from build123d import *

# Parameters (mm, degrees)
SKETCH1_W           = 88.9
SKETCH1_H           = 12.7
BOSS_EXTRUDE1_DEPTH = 6.35
SKETCH2_W           = 14.725
SKETCH2_H           = 6.326510552
SKETCH2_W_2         = 15.361563021
SKETCH2_H_2         = 6.35
BOSS_EXTRUDE2_DEPTH = 19.05
CUT_EXTRUDE1_DEPTH  = 7.35
CUT_EXTRUDE2_DEPTH  = 7.35


with BuildPart() as part:
    # Sketch1 → Boss-Extrude1 (new body)
    with BuildSketch(Plane(origin=(0, 0, 0), x_dir=(1, 0, 0), z_dir=(0, 1, 0))):
        with Locations((44.45, -6.35)):
            Rectangle(SKETCH1_W, SKETCH1_H)
    extrude(amount=BOSS_EXTRUDE1_DEPTH)

    # Sketch2 → Boss-Extrude2 (add)
    with BuildSketch(Plane(origin=(0, 0, 0), x_dir=(-1, 0, 0), z_dir=(0, 0, -1))):
        with Locations((-68.2625, 3.186744724)):
            Rectangle(SKETCH2_W, SKETCH2_H)
        with Locations((-20.95578151, 3.175)):
            Rectangle(SKETCH2_W_2, SKETCH2_H_2)
    extrude(amount=BOSS_EXTRUDE2_DEPTH)

    # Sketch3 → Cut-Extrude1 (cut, through all)
    with BuildSketch(Plane(origin=(0, 6.35, 0), x_dir=(1, 0, 0), z_dir=(0, 1, 0))):
        Polygon((12.7, -6.35), (12.7, -4.1), (0, -4.1), (0, -8.6), (12.7, -8.6), align=None)
        Polygon((76.2, -6.35), (76.2, -4.1), (88.9, -4.1), (88.9, -8.6), (76.2, -8.6), align=None)
    extrude(amount=-CUT_EXTRUDE1_DEPTH, mode=Mode.SUBTRACT)

    # Sketch4 → Cut-Extrude2 (cut, through all)
    with BuildSketch(Plane(origin=(0, 6.35, 0), x_dir=(1, 0, 0), z_dir=(0, 1, 0))):
        Polygon((20.95578151, -12.7), (22.91828151, -12.7), (22.91828151, -6.35), (24.99328151, -6.35), (24.99328151, -3.302), (22.91828151, -3.302), (22.91828151, 12.7), (18.99328151, 12.7), (18.99328151, -3.302), (16.91828151, -3.302), (16.91828151, -6.35), (18.99328151, -6.35), (18.99328151, -12.7), align=None)
        Polygon((70.54328151, 12.7), (70.54328151, -3.302), (72.61828151, -3.302), (72.61828151, -6.35), (70.54328151, -6.35), (70.54328151, -12.7), (68.58078151, -12.7), (66.61828151, -12.7), (66.61828151, -6.35), (64.54328151, -6.35), (64.54328151, -3.302), (66.61828151, -3.302), (66.61828151, 12.7), align=None)
    extrude(amount=-CUT_EXTRUDE2_DEPTH, mode=Mode.SUBTRACT)


solid = part.part
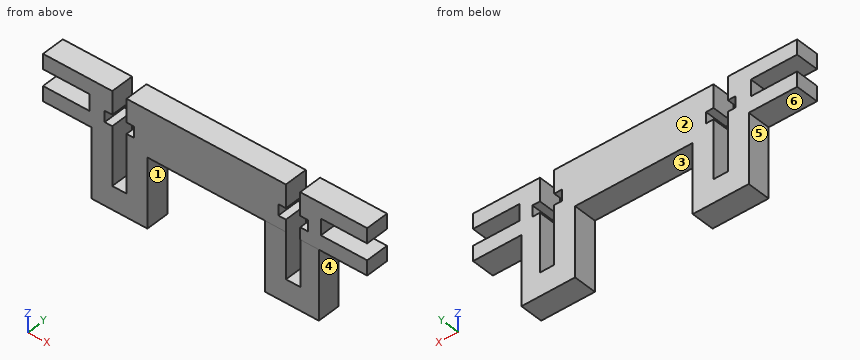
Can you work these out from the model? Positions are in its coordinate system, mm. Face numbers are marked on the shaded views. A direction names the side the tool comes from. Coordinates: 2 decimals unless noted, no trailing zeros. Write each loop counter-clockwise with the first axis right and the second up, starting at its lowest first coordinate (ties: lowest second). Pieces come first, ordered by that corner, then holes. Notation, with made-up numbers: (44.5, 28.25) -> (95.5, 28.25) arc R7 cw to (95.5, 34.25) -> close; hole circle Ø4 at (-32, 10). An arc over 180 degrees is marked (long way). Write item = value, one per line.
(1) Imagine slicing it at B-B (x = 6.5). Please give me the cut outline in (y, z).
Verdict:
outline = (0, 0) -> (6.35, 0) -> (6.35, 4.1) -> (0, 4.1) -> close; (0, 8.6) -> (6.35, 8.6) -> (6.35, 12.7) -> (0, 12.7) -> close
(2) If I drill on probe 1 along X at (y, z) = (2, -4) (3 decimals); probe 2 along X at (y, z) = (3, 4.5); probe 3 along X at (y, z) = (3.25, 9.5), over which ranges is the centre line in solid material (lowest first)?
Verdict:
probe_1 = 13.275 to 18.993, 22.918 to 28.637, 60.9 to 66.618, 70.543 to 75.625
probe_2 = 12.7 to 16.92, 24.99 to 64.54, 72.62 to 76.2
probe_3 = 0 to 18.99, 22.92 to 66.62, 70.54 to 88.9
(3) On a 3-axis mill with a long thin cutter (end or side, diameter ignored), from which of +Z, -Z, +X, -X, +Y, -Y can I reach the whole of each face in a straight line? I mean the marked faces 1 and 2. Say none if no direction works.
Verdict:
face_1 = -Z, +Y, -Y
face_2 = +Z, -Z, +X, -X, +Y
(4) For pin 1 (3 mm diameter, centred on y = 2, z = -8.5, fed in from +X) (3 decimals); pin 2 (1.9 mm diameter, centred on y = 3.5, z = -7.5, fed in from -X) (3 decimals); pin 3 (1 mm diameter, centred on x = 74.5, z = -12.5, fed in from -Y), each with a flat end and sliding along its axis, tell me the tip position at first contact or that it passes through.
Verdict:
pin_1 = 75.625
pin_2 = 13.275
pin_3 = 0.02
(5) Imagine slicing it at C-C (z = -13.5). Please give me the cut outline in (x, y) (3 decimals), and give its area (3 significant figures).
Verdict:
outline = (13.275, 0) -> (28.637, 0) -> (28.637, 6.35) -> (13.275, 6.35) -> close; (60.9, 0.023) -> (75.625, 0.023) -> (75.625, 6.35) -> (60.9, 6.35) -> close
area = 191 mm^2
(6) Imagine slicing it at D-D (x = 36). Please give me the cut outline in (y, z), and give its area (3 significant figures).
Verdict:
outline = (0, 0) -> (6.35, 0) -> (6.35, 12.7) -> (0, 12.7) -> close
area = 80.6 mm^2
(7) Imagine slicing it at A-A (z = -5). Please give me the cut outline in (x, y) (3 decimals), and give its area (3 significant figures).
Verdict:
outline = (13.275, 0) -> (18.993, 0) -> (18.993, 6.35) -> (13.275, 6.35) -> close; (22.918, 0) -> (28.637, 0) -> (28.637, 6.35) -> (22.918, 6.35) -> close; (60.9, 0.023) -> (66.618, 0.023) -> (66.618, 6.35) -> (60.9, 6.35) -> close; (70.543, 0.023) -> (75.625, 0.023) -> (75.625, 6.35) -> (70.543, 6.35) -> close
area = 141 mm^2
(8) Thinking about a two-plate mould opening in X: for the marked faces 3, 4, 5 and 6, which applies, +X half, -X half, draft (parallel to the pull), parting line (faces both ways), or undercut?
Verdict:
face_3 = undercut
face_4 = +X half
face_5 = -X half
face_6 = draft
